Part model, mm, in its own coordinate system. A direction names the side the tool comes from. Give positions to 0.01 mm unless a question says otherwise; leave off trailing zeros. Order: outer loops, then holes, each group sorted by start corner. A loop starts at its lowest first (then second) coordinate and runs counter-clockwise, first axis right, second up. Notation, with made-up numbers: M 53.5,69 L 97.5,69 A12 cw 97.5,80 Z; hole C 60.25,22.25 d10. An arc over 180 degrees is marked long. Write each question's results on one line, items separated by ' | '. Start each with the question number.
from build123d import *

# Parameters (mm, degrees)
FILLET1_R                                  = 3
FILLET2_R                                  = 1
CBORE_FOR_M2_5_SHCS1_D                     = 2.9
CBORE_FOR_M2_5_SHCS1_DEPTH                 = 8
CBORE_FOR_M2_5_SHCS1_CBORE_D               = 5.5
CBORE_FOR_M2_5_SHCS1_CBORE_DEPTH           = 4.5
CBORE_FOR_M2_5_SHCS1_TIP                   = 0.871247898
CBORE_FOR_M2_5_SHCS1_ON_FACE_2_D           = 2.9
CBORE_FOR_M2_5_SHCS1_ON_FACE_2_DEPTH       = 8
CBORE_FOR_M2_5_SHCS1_ON_FACE_2_CBORE_D     = 5.5
CBORE_FOR_M2_5_SHCS1_ON_FACE_2_CBORE_DEPTH = 4.5
CBORE_FOR_M2_5_SHCS1_ON_FACE_2_TIP         = 0.871247898


with BuildPart() as part:
    # Sketch2 → Revolve1 (revolve)
    with BuildSketch(Plane(origin=(0, 0, 0), x_dir=(1, 0, 0), z_dir=(0, 1, 0))):
        Polygon((-23, 2), (-23, 3.5), (-25, 5.5), (-25, 18), (-19, 18), (-19, -2), (-25.3, -2), (-25.3, 0), (-29.5, 0), (-29.5, 6.6), (-27.5, 6.6), (-27.5, 2), align=None)
    revolve(axis=Axis((0, 0, -30.363549001), (0, 0, 1)))

    # Fillet1
    fillet1_edges = [part.edges().sort_by_distance(p)[0] for p in [
        (25, 0, -18),
    ]]
    fillet(fillet1_edges, radius=FILLET1_R)

    # Fillet2
    fillet2_edges = [part.edges().sort_by_distance(p)[0] for p in [
        (25.3, 0, 0),
    ]]
    fillet(fillet2_edges, radius=FILLET2_R)

    # CBORE for M2.5 SHCS1
    with Locations(Plane(origin=(-19.915129246, 15.112499036, -12), x_dir=(-0.604499961451, -0.796605169834, 0), z_dir=(-0.796605169834, 0.604499961451, 0))):
        with Locations((0, 0)):
            CounterBoreHole(CBORE_FOR_M2_5_SHCS1_D / 2, CBORE_FOR_M2_5_SHCS1_CBORE_D / 2, CBORE_FOR_M2_5_SHCS1_CBORE_DEPTH, depth=CBORE_FOR_M2_5_SHCS1_DEPTH)
            with Locations((0, 0, -(CBORE_FOR_M2_5_SHCS1_DEPTH + CBORE_FOR_M2_5_SHCS1_TIP / 2))):  # 118° drill point
                Cone(0, CBORE_FOR_M2_5_SHCS1_D / 2, CBORE_FOR_M2_5_SHCS1_TIP, mode=Mode.SUBTRACT)

    # CBORE for M2.5 SHCS1 on face 2
    with Locations(Plane(origin=(19.915129246, -15.112499036, -12), x_dir=(0.604500067696, 0.79660508921, 0), z_dir=(0.79660508921, -0.604500067696, 0))):
        with Locations((0, 0)):
            CounterBoreHole(CBORE_FOR_M2_5_SHCS1_ON_FACE_2_D / 2, CBORE_FOR_M2_5_SHCS1_ON_FACE_2_CBORE_D / 2, CBORE_FOR_M2_5_SHCS1_ON_FACE_2_CBORE_DEPTH, depth=CBORE_FOR_M2_5_SHCS1_ON_FACE_2_DEPTH)
            with Locations((0, 0, -(CBORE_FOR_M2_5_SHCS1_ON_FACE_2_DEPTH + CBORE_FOR_M2_5_SHCS1_ON_FACE_2_TIP / 2))):  # 118° drill point
                Cone(0, CBORE_FOR_M2_5_SHCS1_ON_FACE_2_D / 2, CBORE_FOR_M2_5_SHCS1_ON_FACE_2_TIP, mode=Mode.SUBTRACT)


solid = part.part
(1) Probe L1, parallel to Y at x = 0, z = -5.75; L2, parallel to Y at x = 0, z = -3.5; L3, parallel to Y at x = -0.5, z = -11 (3 decimals). List the from-to ranges inside material, lowest first.
(2) Pull direction Z, two halves, no side cores. Call faces 1 (the conical face through (17.044, -15.629, -3.625)), 2 (the flat face through (-20, 20, -6.6)), 3 (the cylindrical face through (5.48, 24.7, 1.49)), 4 (the cylindrical face through (17.932, -14.057, -9.273)): +Z half, -Z half, draft (parallel to the pull), parting line (faces both ways), or undercut.
(3) Drop flat-ended pins along their axis: P1, Ø16.5, axis at x = 2.5, y = 8, coming from the -Z side; P2, Ø5, axis at x = -5.5, z = -15, coming from the -Y side; P3, Ø4, axis at x = 18.5, z = -0.5, coming from the +Y side; P4, Ø8, axis at x = 8, z = -7.5, coming from the -Y side. Give the stop position or say it passes through.
(4) Tool access for faces 5 (the cylindrical face through (5.961, 26.846, -4.268)), 6 (the flat face through (-26.4, 2, 0)), 7 (the flat face through (17.046, -11.449, -13.184)), 8 (the cylindrical face through (-28.14, -8.86, -3.35)): list every direction of +Z, -Z, +X, -X, +Y, -Y with a clear straight run to the whole face (end or side of a thin tool).
(5) Saw through at A-A on x = 0. Give the cut face in (y, z), plus the area to 3 significant figures.
Taken from the geometry:
1) L1: y = -29.5 to -27.5, -25 to -19, 19 to 25, 27.5 to 29.5 | L2: y = -29.5 to -27.5, -23 to -19, 19 to 23, 27.5 to 29.5 | L3: y = -24.995 to -18.993, 18.993 to 24.995
2) face 1: undercut | face 2: -Z half | face 3: draft | face 4: undercut
3) P1: passes through | P2: stops at y = -24.82 | P3: stops at y = 24.45 | P4: stops at y = -29.21
4) face 5: -Z | face 6: +Z | face 7: none | face 8: +Z, -Z
5) outline: M -29.5,-6.6 L -27.5,-6.6 L -27.5,-2 L -23,-2 L -23,-3.5 L -25,-5.5 L -25,-15 A3 ccw -22,-18 L -19,-18 L -19,2 L -25.3,2 L -25.3,1 A1 cw -26.3,0 L -29.5,0 Z; M 19,-18 L 22,-18 A3 ccw 25,-15 L 25,-5.5 L 23,-3.5 L 23,-2 L 27.5,-2 L 27.5,-6.6 L 29.5,-6.6 L 29.5,0 L 26.3,0 A1 cw 25.3,1 L 25.3,2 L 19,2 Z | area: 264 mm²
